Print and shaded views of the part. All mm, measured from the part's lowest x, y and z. A direction names the side the tool comes from. Give positions to 0.01 mm unless a question says otherwise; leave off trailing zeros. Loops run counter-clockwise (first coordinate to the right, second up) from the corner with the lowest first, then second, coordinate; pieces in that order, holes last. Notation, with made-up numbers: M 26.5,55.25 L 64.5,55.25 A23 cw 64.5,92.25 Z; hole C 19.5,-8.75 d11. An arc over 180 degrees is marked long. Put each result on its own line as item: value. Start each with the question number.
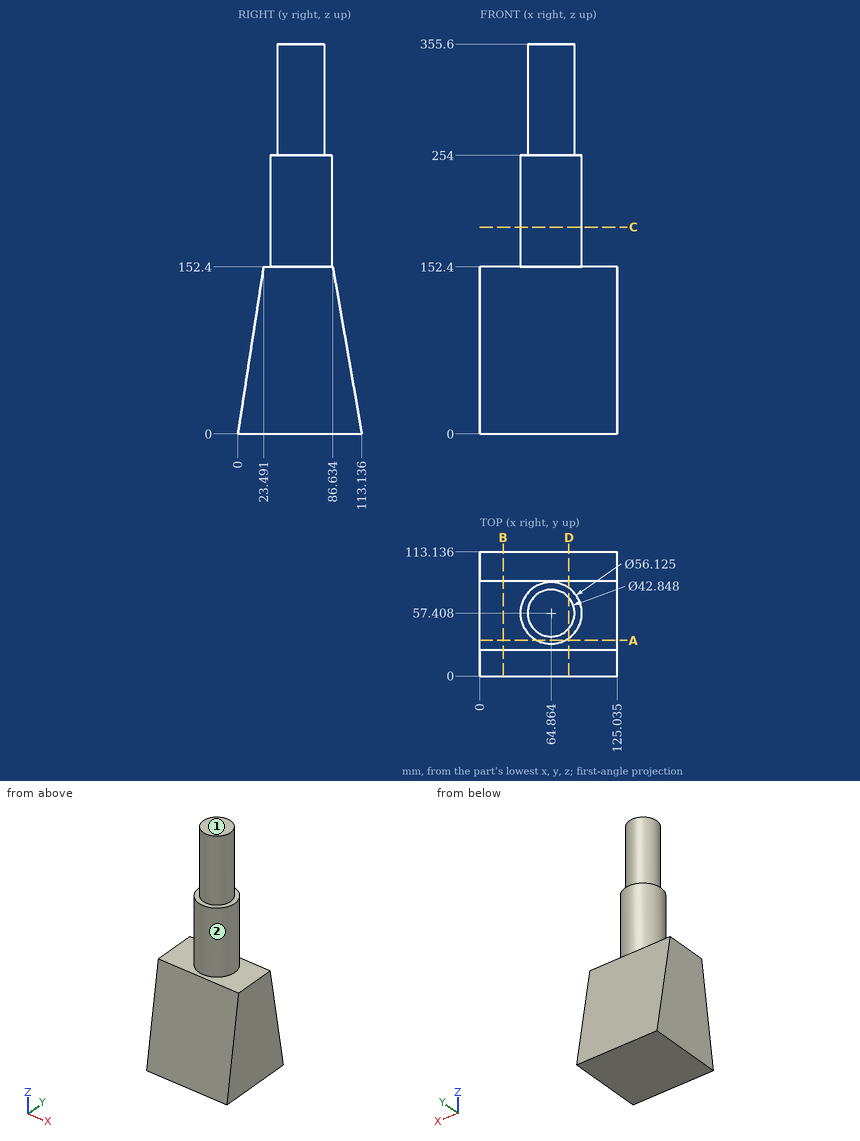
1) Wall check: L1, parallel to Z at x = 22, y = 27.5; L2, parallel to Z at x = 61, y = 81; L3, parallel to Y at x = 72.5, z = 320 (1 decimal). Give the ranges that are in metal, low to high.
2) Band-saw the part on B-B on x = 21. Give the cut face in (y, z) (1 decimal).
3) Which spindle directions (+Z, -Z, +X, -X, +Y, -Y) get a long thin tool onto all of the face, cutting with end or side? Do the marked faces 1 and 2. Say none if no direction does.
4) Pin check, flat tips, straight feed: pin 1 Ø6 at (x, z) = (61.5, 143) entering from -Y; pin 2 Ø8 at (x, z) = (51.5, 94) entering from +Y (1 decimal); pin 3 Ø10 at (x, z) = (78.5, 117.5) entering from -Y. Stop position of each tip, or through.
5) Band-saw the part on A-A on y = 32.5. Give the cut face in (x, z) (1 decimal).
6) Band-saw the part on D-D on x = 81. Give the cut face in (y, z) (1 decimal).
7) Band-saw the part on C-C on z = 188.5. Give the cut face in (x, y) (1 decimal), then the cut area to 3 significant figures.
Evaluation:
1. L1: 0 to 152.4
1. L2: 0 to 254
1. L3: 37.4 to 77.4
2. outline: M 0,0 L 113.1,0 L 86.6,152.4 L 23.5,152.4 Z
3. face 1: +Z, +X, -X, +Y, -Y
3. face 2: +Z
4. pin 1: y = 21.58
4. pin 2: y = 97.5
4. pin 3: y = 17.34
5. outline: M 0,0 L 125,0 L 125,152.4 L 77.8,152.4 L 77.8,254 L 51.9,254 L 51.9,152.4 L 0,152.4 Z
6. outline: M 0,0 L 113.1,0 L 86.6,152.4 L 80.4,152.4 L 80.4,254 L 71.5,254 L 71.5,355.6 L 43.3,355.6 L 43.3,254 L 34.4,254 L 34.4,152.4 L 23.5,152.4 Z
7. outline: C 64.9,57.4 d56.1
7. area: 2,470 mm2
